Source: three-view drawing plus pictorial views. Frame: mm from the lowest corner of the part. A direction names the side the tool comes from. Coordinates: 2 decimals unless noted, no trailing zeros. Write each loop counter-clockwise with the first axis right and the second up, starting at its lowest first coordinate (ties: lowest second). Pieces come first, ordered by that corner, then holes. Notation, with made-up numbers: (37, 47) -> (48, 47) arc R26 ccw to (48, 65) -> close; hole circle Ø1 at (2, 66.5). An arc over 180 degrees is marked (long way). One line per question, with ' | ' between items. Start each with the question number.
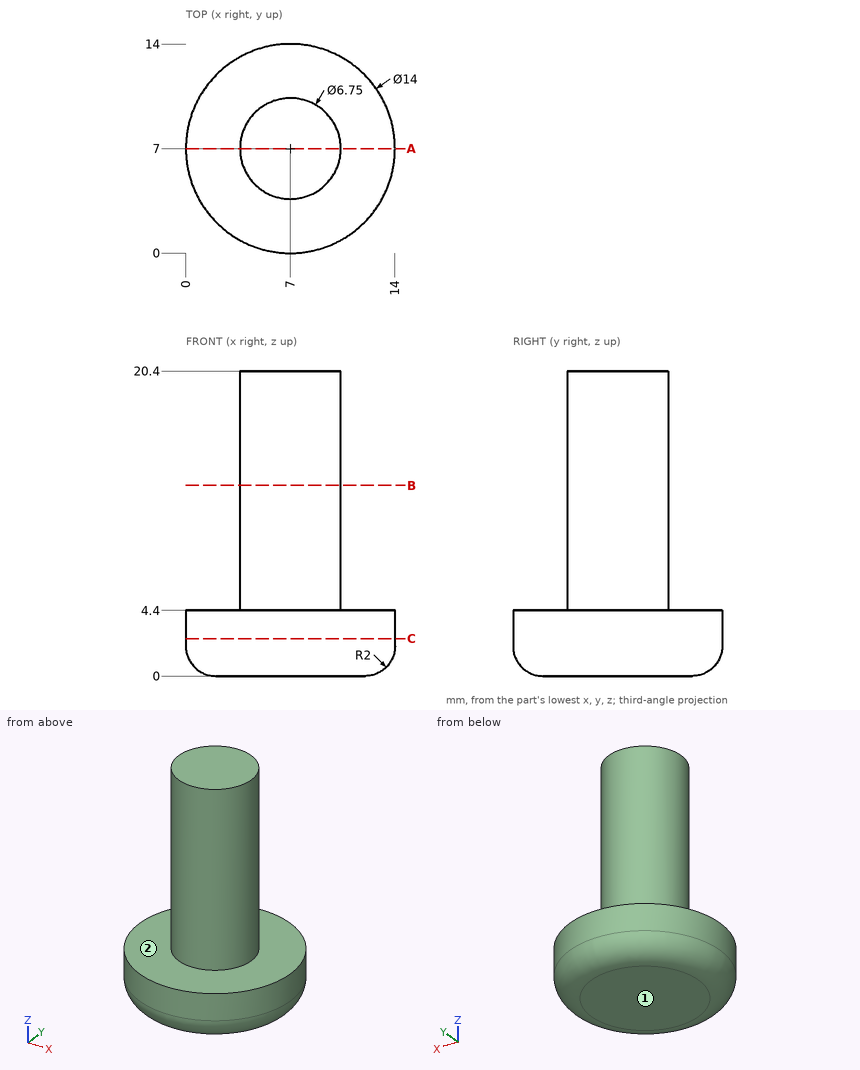
1) Section C-C, the plane z = 2.5. Return loops of the section in (x, y).
2) Section A-A, the plane y = 7. Return loops of the section in (x, z) (3 decimals), then the cut area to 3 significant figures.
3) Ray query, line 1 (Z direction, x = 11.5, y = 5.5); line 2 (X direction, y = 8.5, z = 13.25); line 3 (Z direction, x = 3.25, y = 2.75). Return the intervals inside material, ascending.
4) Access query for the marked faces 1 and 2. Directions: +Z, -Z, +X, -X, +Y, -Y. A direction counts if a zero-diameter tool reaches every point of the face in a straight line with its end or side. Return the directions, or none.
5) Section B-B, the plane z = 12.75. Return loops of the section in (x, y) (3 decimals), then the cut area to 3 significant figures.
6) First-contact query: P1, Ø1.5, axis at y = 8.5, z = 7.5, coming from the +X side; P2, Ø2, axis at x = 2, z = 9, coming from the -Y side; P3, Ø1.5, axis at x = 3.5, z = 9.5, coming from the -Y side; P4, Ø5, axis at x = 9, z = 9.5, coming from the +Y side (3 decimals). Flat tips, straight axial feed; report the tip coordinate or a pass-through.
Answer block:
1) outline: circle Ø14 at (7, 7)
2) outline: (0, 2) arc R2 ccw to (2, 0) -> (12, 0) arc R2 ccw to (14, 2) -> (14, 4.4) -> (10.375, 4.4) -> (10.375, 20.4) -> (3.625, 20.4) -> (3.625, 4.4) -> (0, 4.4) -> close | area: 168 mm2
3) line 1: z = 0 to 4.4 | line 2: x = 3.98 to 10.02 | line 3: z = 0.11 to 4.4
4) face 1: -Z, +X, -X, +Y, -Y | face 2: +Z
5) outline: circle Ø6.75 at (7, 7) | area: 35.8 mm2
6) P1: stops at x = 10.29 | P2: passes through | P3: stops at y = 5.04 | P4: stops at y = 10.375
